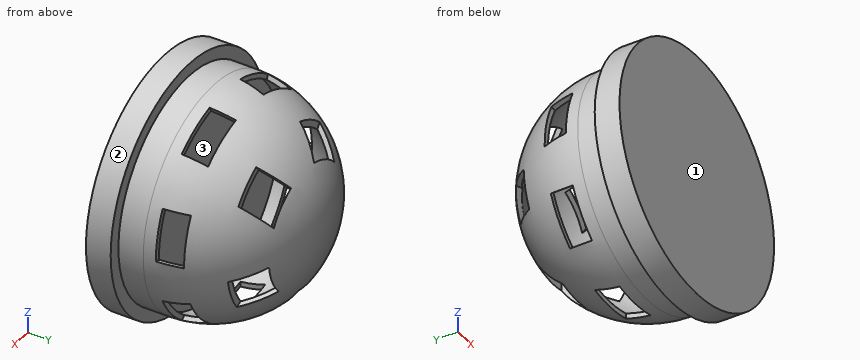
from build123d import *

# Parameters (mm, degrees)
SCHIZZO1_R                   = 50
ESTRUSIONE_ESTRUSIONE1_DEPTH = 10
SCHIZZO2_R                   = 45
ESTRUSIONE_ESTRUSIONE2_DEPTH = 10
SCHIZZO14_W                  = 20
SCHIZZO14_H                  = 10
TAGLIO_ESTRUSIONE2_DEPTH     = 53
RIPETIZIONECIRCOLARE6_COUNT  = 7
SCHIZZO17_W                  = 15
SCHIZZO17_H                  = 10
TAGLIO_ESTRUSIONE3_DEPTH     = 53
RIPETIZIONECIRCOLARE7_COUNT  = 5


with BuildPart() as part:
    # Schizzo1 → Estrusione-Estrusione1 (new body)
    with BuildSketch(Plane(origin=(0, 0, 0), x_dir=(1, 0, 0), z_dir=(0, 1, 0))):
        with Locations(Location((0, 0, 0), (0, 0, 270))):
            Circle(SCHIZZO1_R)
    extrude(amount=ESTRUSIONE_ESTRUSIONE1_DEPTH)

    # Schizzo2 → Estrusione-Estrusione2 (add)
    with BuildSketch(Plane(origin=(0, 10, 0), x_dir=(1, 0, 0), z_dir=(0, 1, 0))):
        with Locations(Location((0, 0, 0), (0, 0, 270))):
            Circle(SCHIZZO2_R)
    extrude(amount=ESTRUSIONE_ESTRUSIONE2_DEPTH)

    # Schizzo6 → Rivoluzione9 (revolve)
    with BuildSketch(Plane(origin=(0, 0, 0), x_dir=(0, 0, -1), z_dir=(1, 0, 0)), mode=Mode.PRIVATE) as rivoluzione9_sk:
        with BuildLine():
            Line((0, 65), (0, 63))
            ThreePointArc((0, 63), (-30.405591591, 50.405591591), (-43, 20))
            Line((-43, 20), (-45, 20))
            ThreePointArc((-45, 20), (-31.819805153, 51.819805153), (0, 65))
        make_face()
    revolve(rivoluzione9_sk.sketch.rotate(Axis((0, 119.686269666, 0), (0, -1, 0)), 180), axis=Axis((0, 119.686269666, 0), (0, -1, 0)))

    # Schizzo14 → Taglio-Estrusione2 (cut)
    with BuildSketch(Plane.XY):
        with Locations((0, 29.930993036)):
            Rectangle(SCHIZZO14_W, SCHIZZO14_H)
    taglio_estrusione2 = extrude(amount=-TAGLIO_ESTRUSIONE2_DEPTH, mode=Mode.SUBTRACT)

    # RipetizioneCircolare6: Taglio-Estrusione2 ×7 about axis
    ripetizionecircolare6_axis = Axis((0, 0, 0), (0, 1, 0))
    for i in range(1, RIPETIZIONECIRCOLARE6_COUNT):
        add(taglio_estrusione2.rotate(ripetizionecircolare6_axis, i * 360 / RIPETIZIONECIRCOLARE6_COUNT), mode=Mode.SUBTRACT)

    # Schizzo17 → Taglio-Estrusione3 (cut)
    with BuildSketch(Plane.XY):
        with Locations((-2.5, 52.858470441)):
            Rectangle(SCHIZZO17_W, SCHIZZO17_H)
    taglio_estrusione3 = extrude(amount=-TAGLIO_ESTRUSIONE3_DEPTH, mode=Mode.SUBTRACT)

    # RipetizioneCircolare7: Taglio-Estrusione3 ×5 about axis
    ripetizionecircolare7_axis = Axis((0, 0, 0), (0, 1, 0))
    for i in range(1, RIPETIZIONECIRCOLARE7_COUNT):
        add(taglio_estrusione3.rotate(ripetizionecircolare7_axis, i * 360 / RIPETIZIONECIRCOLARE7_COUNT), mode=Mode.SUBTRACT)


solid = part.part
Verification items for the finished model (mm, model axes). Face numbers are marked on the shaded views. Coordinates: 2 decimals unless noted, no trailing zeros. Loops run counter-clockwise (first coordinate to the right, second up) from the corner with the lowest first, then second, coordinate; pieces in that order, holes last. Notation, with made-up numbers: (-13.5, 20) -> (16.5, 20) arc R32 ccw to (16.5, 53) -> close; hole circle Ø9 at (84.25, -14). An arc over 180 degrees is marked (long way). Answer as a JSON object with one key per item and string values. Group by question number.
Item 1: Depth check by flat-ended pin: pin 1 (11.5 mm diameter, centred on x = 20.5, z = 37.5, fed in from +Y); pin 2 (12 mm diameter, centred on y = 19.5, z = 12.5, fed in from -X); pin 3 (5 mm diameter, centred on x = -31.5, z = -5, fed in from +Y); pin 4 (5 mm diameter, centred on x = -34.5, z = 34, fed in from -Y). Enter the tip coordinate at first touch or a pass-through.
Item 2: Sectioned sample at C-C on z = 38. Record the boundary of the cut face in (x, y).
Item 3: Sectioned sample at B-B on x = 0. Record the boundary of the cut face in (y, z).
Item 4: Scan lines: probe 1 along Y at (x, z) = (26.5, -42); probe 2 along Z at (x, y) = (-22, 24.5); probe 3 along X at (y, z) = (32.5, 28). Record each from-to range of solid material in increasing order.
Item 5: Mould release check, pull along Z, two halves, no side actions. Record for the marked faces 1, 2 and 3: +Z half, -Z half, draft (parallel to the pull), parting line (faces both ways), or undercut.
Item 6: Sectioned sample at A-A on y = 31. Record the boundary of the cut face in (x, z).
Item 7: Sectioned sample at D-D on y = 5. Record the boundary of the cut face in (x, z).
Evaluation:
{
 "1": {"pin 1": "stops at y = 45.63", "pin 2": "stops at x = -44.53", "pin 3": "stops at y = 47.86", "pin 4": "stops at y = 0"},
 "2": {"outline": "(-32.5, 0) -> (32.5, 0) -> (32.5, 10) -> (24.1, 10) -> (24.1, 20) arc R24.1 ccw to (23.59, 24.93) -> (19.51, 24.93) arc R20.12 cw to (20.12, 20) -> (-20.12, 20) arc R20.12 cw to (-19.51, 24.93) -> (-23.59, 24.93) arc R24.1 ccw to (-24.1, 20) -> (-24.1, 10) -> (-32.5, 10) -> close; (-18.92, 34.93) -> (-13.49, 34.93) arc R20.12 cw to (13.49, 34.93) -> (18.92, 34.93) arc R24.1 ccw to start"},
 "3": {"outline": "(0, -50) -> (10, -50) -> (10, -45) -> (20, -45) arc R45 ccw to (24.93, -44.73) -> (24.93, -42.72) arc R43 cw to (20, -43) -> (20, 43) arc R43 cw to (57.86, -20.39) -> (57.86, -24.33) arc R45 ccw to (20, 45) -> (10, 45) -> (10, 50) -> (0, 50) -> close; (34.93, -42.45) arc R45 ccw to (47.86, -35.34) -> (47.86, -32.76) arc R43 cw to (34.93, -40.32) -> close"},
 "4": {"probe 1": "y = 0 to 10", "probe 2": "z = -39 to -36.67, 36.67 to 39", "probe 3": "x = -32.94 to -30.15, 30.15 to 32.94"},
 "5": {"face 1": "draft", "face 2": "parting line", "face 3": "undercut"},
 "6": {"outline": "(-43.63, -0.3) arc R43.63 ccw to (-39.44, -18.66) -> (-37.78, -17.34) arc R41.57 cw to (-41.56, -0.77) -> close; (-39.18, 19.2) -> (-37.11, 18.73) arc R41.57 cw to (-26.52, 32.01) -> (-27.44, 33.93) arc R43.63 ccw to start; (-26.97, -34.3) arc R43.63 ccw to (-10, -42.47) -> (-10, -40.35) arc R41.57 cw to (-25.31, -32.98) -> close; (-9.42, 42.61) -> (-8.5, 40.69) arc R41.57 cw to (8.5, 40.69) -> (9.42, 42.61) arc R43.63 ccw to start; (10, -42.47) arc R43.63 ccw to (26.97, -34.3) -> (25.31, -32.98) arc R41.57 cw to (10, -40.35) -> close; (26.52, 32.01) arc R41.57 cw to (37.11, 18.73) -> (39.18, 19.2) arc R43.63 ccw to (27.44, 33.93) -> close; (37.78, -17.34) -> (39.44, -18.66) arc R43.63 ccw to (43.63, -0.3) -> (41.56, -0.77) arc R41.57 cw to start"},
 "7": {"outline": "circle Ø100 at (0, 0)"}
}
